Design review of the part built by this model. Coordinates are the model's own, in mm. A direction names the side the tool comes from. Give positions to 0.01 mm unless a question says otherwise; leave off trailing zeros. Write each loop counter-clockwise with the first axis right and the second up, starting at its lowest first coordinate (ties: lowest second). Pieces come first, ordered by that corner, then holes. Notation, with made-up numbers: M 53,64.25 L 74,64.25 A13 cw 74,72.25 Z; hole C 20.5,68 d1. An arc over 180 degrees is marked long. One line per item, written item: value. Start each with the question number.
```python
from build123d import *

# Parameters (mm, degrees)
BOSS_EXTRUDE1_DEPTH     = 15
FILLET1_R               = 5
CUT_EXTRUDE3_DEPTH      = 1.2
CUT_EXTRUDE4_DEPTH      = 35.323825544
CUT_EXTRUDE4_DEPTH_BACK = 10
FILLET2_R               = 3
FILLET3_R               = 3
FILLET4_R               = 5
FILLET5_R               = 2


with BuildPart() as part:
    # Sketch1 → Boss-Extrude1 (new body)
    with BuildSketch(Plane.XY):
        Polygon((0, 0), (0, 4), (-5, 4), (-5, -5), (10, -5), (10, 12.5), (5, 17.5), (-11, 17.5), (-15, 17.5), (-15, 7.5), (-11, 7.5), (-11, 12.5), (5, 12.5), (5, 0), align=None)
    extrude(amount=BOSS_EXTRUDE1_DEPTH)

    # Fillet1
    fillet1_edges = [part.edges().sort_by_distance(p)[0] for p in [
        (5, 12.5, 7.5),
    ]]
    fillet(fillet1_edges, radius=FILLET1_R)

    # Sketch2 → Cut-Extrude3 (cut)
    with BuildSketch(Plane(origin=(11.25, 11.25, 0), x_dir=(0, 0, -1), z_dir=(0.7071067811865487, 0.7071067811865465, 0))):
        with BuildLine():
            Line((-8.6, 7.503300859), (-6.4, 7.503300859))
            ThreePointArc((-6.4, 7.503300859), (-5.339339828, 7.063961031), (-4.9, 6.003300859))
            Line((-4.9, 6.003300859), (-4.9, 4.603300859))
            ThreePointArc((-4.9, 4.603300859), (-5.339339828, 3.542640687), (-6.4, 3.103300859))
            Line((-6.4, 3.103300859), (-8.6, 3.103300859))
            ThreePointArc((-8.6, 3.103300859), (-9.660660172, 3.542640687), (-10.1, 4.603300859))
            Line((-10.1, 4.603300859), (-10.1, 6.003300859))
            ThreePointArc((-10.1, 6.003300859), (-9.660660172, 7.063961031), (-8.6, 7.503300859))
        make_face()
    extrude(amount=-CUT_EXTRUDE3_DEPTH, mode=Mode.SUBTRACT)

    # Sketch2<5> → Cut-Extrude4 (cut, two sides: drawn at the far end of the back side and taken through both)
    with BuildSketch(Plane(origin=(11.25, 11.25, 0), x_dir=(0, 0, -1), z_dir=(0.7071067811865487, 0.7071067811865465, 0)).offset(-CUT_EXTRUDE4_DEPTH_BACK)):
        with BuildLine():
            Line((-9, 3.157617629), (-9, 7.448984088))
            ThreePointArc((-9, 7.448984088), (-9.793733639, 6.911595965), (-10.1, 6.003300859))
            Line((-10.1, 6.003300859), (-10.1, 4.603300859))
            ThreePointArc((-10.1, 4.603300859), (-9.793733639, 3.695005753), (-9, 3.157617629))
        make_face()
        with BuildLine():
            ThreePointArc((-4.9, 6.003300859), (-5.206266361, 6.911595965), (-6, 7.448984088))
            Line((-6, 7.448984088), (-6, 3.157617629))
            ThreePointArc((-6, 3.157617629), (-5.206266361, 3.695005753), (-4.9, 4.603300859))
            Line((-4.9, 4.603300859), (-4.9, 6.003300859))
        make_face()
    extrude(amount=CUT_EXTRUDE4_DEPTH + CUT_EXTRUDE4_DEPTH_BACK, mode=Mode.SUBTRACT)

    # Fillet2
    fillet2_edges = [part.edges().sort_by_distance(p)[0] for p in [
        (0, 4, 7.5),
    ]]
    fillet(fillet2_edges, radius=FILLET2_R)

    # Fillet3
    # the kernel refuses this fillet: 3 mm, written as the material it takes off along each edge
    with BuildSketch(Plane(origin=(-5, 4, -7.071067812), x_dir=(1, 0, 0), z_dir=(0, 0, 1))) as fillet3_piece_1:
        with BuildLine():
            CenterArc((3, -2.828427125), FILLET3_R, 109.471220634, 70.528779366)
            Line((0, -2.828427125), (-0.06, -2.828427125))
            Line((-0.06, -2.828427125), (-0.06, 0))
            Line((-0.06, 0), (0, 0.06))
            ThreePointArc((0, 0.06), (1, 0.06), (1.98, 0.056568542))
            Line((1.98, 0.056568542), (2, 0))
        make_face()
    extrude(amount=29.142135624, mode=Mode.SUBTRACT)

    # Fillet4
    fillet4_edges = [part.edges().sort_by_distance(p)[0] for p in [
        (-15, 17.5, 7.5),
    ]]
    fillet(fillet4_edges, radius=FILLET4_R)

    # Fillet5
    fillet5_edges = [part.edges().sort_by_distance(p)[0] for p in [
        (-11, 12.5, 7.5),
    ]]
    fillet(fillet5_edges, radius=FILLET5_R)


solid = part.part
```
Q1. Take a section at C-C, the plane z = 13. Give the boundary of the cut face in (x, y), then the cut area to 3 significant figures.
Q2. The part is to be moulded in two halves that separate along Y. For faces 1 (the face through (9.2, 13.3, 7.4)), 2 (the face through (-5, -2, 7)), 3 (the face through (6.429, 11.704, 5.181)), say which applies: pulls with the +Y half, pulls with the -Y half, needs draft (parallel to the pull), parting line crosses it, or undercut.
Q3. Take a section at A-A, the plane y = 0.5. Give the boundary of the cut face in (x, z).
Q4. Wall thickness on line 1 (Y direction, x = 2.75, z = 5.5); line 2 (X direction, y = 6.75, z = 13.5); line 3 (X direction, y = 11.25, z = 1.5): over which ranges is each line inside the solid? List them lowest first. Write a range as from..to.
Q5. For P1, Ø8, axis at y = 1.5, z = 5, coming from the -X side; P2, Ø6, axis at x = -2, y = 13.5, coming from the -Z side; P3, Ø4.5, axis at x = -14, z = 5.5, coming from the -Y side, all flat-tipped, find the tip position at first contact; note any pin that passes through.
Q6. Take a section at B-B, the plane x = 0.5. Give the boundary of the cut face in (y, z), then the cut area to 3 significant figures.
Q7. Machinability: for faces 4 (the face through (-10.43, 11.9, 7.6)), 5 (the face through (3.5, 11.07, 7.6)), 6 (the face through (5, 12, 6)), which of the approach directions +Z, -Z, +X, -X, +Y, -Y give a long, thin tool a straight path to every point of the face, cutting with its end or side? Answer none if there is none.
Q8. Take a section at D-D, the plane z = 5.25. Give the boundary of the cut face in (x, y), then the cut area to 3 significant figures.
Results list:
1. outline: M -15,7.5 L -11,7.5 L -11,10.5 A2 cw -9,12.5 L 0,12.5 A5 cw 5,7.5 L 5,0 L 0,0 L 0,1 A3 ccw -3,4 A3 ccw -5,1.17 L -5,-5 L 10,-5 L 10,12.5 L 5,17.5 L -10,17.5 A5 ccw -15,12.5 Z
1. area: 287 mm^2
2. face 1: pulls with the +Y half
2. face 2: needs draft
2. face 3: undercut
3. outline: M -5,0 L 0,0 L 0,15 L -5,15 Z; M 5,0 L 10,0 L 10,15 L 5,15 Z
4. line 1: y = -5..0, 12.94..17.5
4. line 2: x = 5..10
4. line 3: x = -15..-10.85, 3.31..10
5. P1: stops at x = -5
5. P2: stops at z = 0
5. P3: stops at y = 7.5
6. outline: M -5,0 L 0,0 L 0,15 L -5,15 Z; M 12.47,0 L 17.5,0 L 17.5,15 L 12.47,15 Z
6. area: 150 mm^2
7. face 4: +Z, -Z, -Y
7. face 5: +Z, -Z
7. face 6: none
8. outline: M -15,7.5 L -11,7.5 L -11,10.5 A2 cw -9,12.5 L 0,12.5 A5 cw 2.16,12.01 L 6.32,16.18 L 5,17.5 L -10,17.5 A5 ccw -15,12.5 Z; M -5,-5 L 10,-5 L 10,12.5 L 8.68,13.82 L 4.51,9.66 A5 cw 5,7.5 L 5,0 L 0,0 L 0,1 A3 ccw -3,4 A3 ccw -5,1.17 Z
8. area: 268 mm^2
